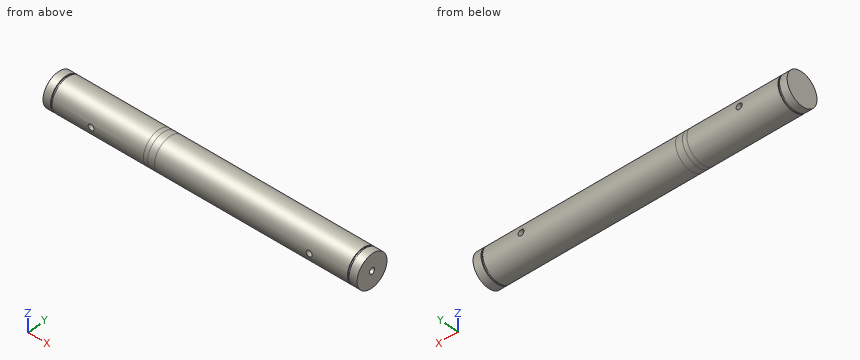
```python
from build123d import *

# Parameters (mm, degrees)
M8_GEWINDEBOHRUNG1_D          = 6.8
M8_GEWINDEBOHRUNG1_DEPTH      = 325
M8_GEWINDEBOHRUNG1_TIP        = 2.042926105
SKIZZE18_W                    = 3.4
SKIZZE18_H                    = 27
M8_GEWINDEBOHRUNG3_AT_2_COUNT = 2
M8_GEWINDEBOHRUNG3_AT_2_PITCH = 250
SPIEGELN2_COPY_1_SKETCH_W     = 3.4
SPIEGELN2_COPY_1_SKETCH_H     = 27
SKIZZE19_W                    = 1.85
SKIZZE19_H                    = 1
SKIZZE20_W                    = 1.85
SKIZZE20_H                    = 1
SKETCH1_W                     = 21.407583332
SKETCH1_H                     = 15.084330907


with BuildPart() as part:
    # Skizze1 → Rotation1 (revolve)
    with BuildSketch(Plane.XY, mode=Mode.PRIVATE) as rotation1_sk:
        Polygon((180, 19), (180, 0), (-180, 0), (-180, 19), (-65, 19), (-65, 27), (-60, 27), (-60, 19.0001), (90, 19.0001), align=None)
    revolve(rotation1_sk.sketch.rotate(Axis((180, 0, 0), (-1, 0, 0)), 90), axis=Axis((180, 0, 0), (-1, 0, 0)))

    # M8 Gewindebohrung1
    with Locations(Plane(origin=(180, 0, 0), x_dir=(0, 0, -1), z_dir=(1, 0, 0))):
        with Locations((0, 0)):
            Hole(M8_GEWINDEBOHRUNG1_D / 2, depth=M8_GEWINDEBOHRUNG1_DEPTH)
            with Locations((0, 0, -(M8_GEWINDEBOHRUNG1_DEPTH + M8_GEWINDEBOHRUNG1_TIP / 2))):  # 118° drill point
                Cone(0, M8_GEWINDEBOHRUNG1_D / 2, M8_GEWINDEBOHRUNG1_TIP, mode=Mode.SUBTRACT)

    # Skizze18 → M8 Gewindebohrung3 (revolve, cut)
    with BuildSketch(Plane(origin=(-125, 0, 0), x_dir=(0, 0, -1), z_dir=(1, 0, 0))):
        with Locations((1.7, 13.5)):
            Rectangle(SKIZZE18_W, SKIZZE18_H)
    m8_gewindebohrung3 = revolve(axis=Axis((-125, -6.35, 0), (0, 1, 0)), mode=Mode.SUBTRACT)

    # M8 Gewindebohrung3 at 2: M8 Gewindebohrung3 ×2
    with Locations(*[(i * M8_GEWINDEBOHRUNG3_AT_2_PITCH, 0, 0) for i in range(1, M8_GEWINDEBOHRUNG3_AT_2_COUNT)]):
        add(m8_gewindebohrung3, mode=Mode.SUBTRACT)

    # Spiegeln2: M8 Gewindebohrung3 across plane
    add(m8_gewindebohrung3.mirror(Plane.ZX), mode=Mode.SUBTRACT)

    # Spiegeln2 copy 1 sketch → Spiegeln2 copy 1 (revolve, cut)
    with BuildSketch(Plane(origin=(125, 0, 0), x_dir=(0, 0, -1), z_dir=(1, 0, 0))):
        with Locations((1.7, -13.5)):
            Rectangle(SPIEGELN2_COPY_1_SKETCH_W, SPIEGELN2_COPY_1_SKETCH_H)
    revolve(axis=Axis((125, 6.35, 0), (0, 1, 0)), mode=Mode.SUBTRACT)

    # Skizze19 → Schnitt-Rotation1 (revolve, cut)
    with BuildSketch(Plane.XY, mode=Mode.PRIVATE) as schnitt_rotation1_sk:
        with Locations((169.825, 18.5)):
            Rectangle(SKIZZE19_W, SKIZZE19_H)
    revolve(schnitt_rotation1_sk.sketch.rotate(Axis((-88.99, 0, 0), (1, 0, 0)), 270), axis=Axis((-88.99, 0, 0), (1, 0, 0)), mode=Mode.SUBTRACT)

    # Skizze20 → Schnitt-Rotation2 (revolve, cut)
    with BuildSketch(Plane.XY, mode=Mode.PRIVATE) as schnitt_rotation2_sk:
        with Locations((-170.475, 18.5)):
            Rectangle(SKIZZE20_W, SKIZZE20_H)
    revolve(schnitt_rotation2_sk.sketch.rotate(Axis((-88.99, 0, 0), (1, 0, 0)), 270), axis=Axis((-88.99, 0, 0), (1, 0, 0)), mode=Mode.SUBTRACT)

    # Sketch1 → Cut-Revolve1 (revolve, cut)
    with BuildSketch(Plane.XY, mode=Mode.PRIVATE) as cut_revolve1_sk:
        with Locations((-62.803513507, 26.542265454)):
            Rectangle(SKETCH1_W, SKETCH1_H)
    revolve(cut_revolve1_sk.sketch.rotate(Axis((-202.232213843, 0, 0), (1, 0, 0)), 270), axis=Axis((-202.232213843, 0, 0), (1, 0, 0)), mode=Mode.SUBTRACT)


solid = part.part
```
Model file for the job. Use its own axes, mm. Coordinates: 2 decimals unless noted, no trailing zeros. Order: outer loops, then holes, each group sorted by start corner. A loop starts at its lowest first (then second) coordinate and runs counter-clockwise, first axis right, second up. Notation, with made-up numbers: (75.25, -37.75) -> (85.25, -37.75) arc R31 cw to (85.25, -2.75) -> close; hole circle Ø11 at (-18, 20). An arc over 180 degrees is marked (long way). Answer as a JSON object with one key per item and string values. Group by question number.
1) Cut at A-A, the plane y = 12. Count the separate pieces of the cut face and the enclosed holes in it, then the cut area to 3 significant figures.
2) Flat gauge pins, fed straight in: pin 1 (4 mm diameter, centred on x = -58, z = -3, fed in from +Y); pin 2 (6 mm diameter, centred on x = -33, y = -8, fed in from -Z); pin 3 (1 mm diameter, centred on x = 24.5, y = 14, fed in from +Z). Where does each tip first touch, or does it go through?
3) Drill centre lines: L1, parallel to X at y = -4.25, z = 0; L2, parallel to Y at x = 137, z = 0. Where is each one in solid material? Low to high.
4) Cut at C-C, the plane x = 30. Write the cut outline in (y, z), then the cut area to 3 significant figures.
Check values:
{
 "1": {"separate pieces": "1", "enclosed holes": "2", "area": "10,500 mm²"},
 "2": {"pin 1": "stops at y = 18.97", "pin 2": "stops at z = -18.33", "pin 3": "stops at z = 13.37"},
 "3": {"L1": "x = -180 to -128.4, -121.6 to 121.6, 128.4 to 180", "L2": "y = -19 to -3.4, 3.4 to 19"},
 "4": {"outline": "circle Ø38 at (0, 0); hole circle Ø6.8 at (0, 0)", "area": "1,100 mm²"}
}
